```python
from build123d import *

# Parameters (mm, degrees)
F1_DEPTH = 24.13
F2_W     = 15.685529
F2_H     = 20.463388
F3_DEPTH = 11.43
F5_DEPTH = 25.146


with BuildPart() as f1:
    # F0 (on Right) → F1 (new body)
    with BuildSketch(Plane.YZ):
        Polygon((0, 21.47734), (-69.962664, 21.47734), (-69.962664, 2.857499), (-33.644756, 2.857499), (0, 2.857499), align=None)
        Polygon((-33.644756, 2.857499), (-69.962664, 2.857499), (-87.845083, 2.857499), (-87.845083, -17.605888), (-33.644756, -17.605888), align=None)
    extrude(amount=F1_DEPTH)

    # F2 (on Right) → F3 (cut)
    with BuildSketch(Plane.YZ):
        with Locations((-7.842764, 12.16742)):
            Rectangle(F2_W, F2_H)
    extrude(amount=F3_DEPTH, mode=Mode.SUBTRACT)

    # F4 (on Right) → F5 (join)
    with BuildSketch(Plane.YZ):
        Polygon((-0.056833, 21.314132), (-70.019497, 21.314132), (-70.019497, 2.694292), (-33.701589, 2.694292), (-0.056833, 2.694292), align=None)
        Polygon((-33.701589, 2.694292), (-70.019497, 2.694292), (-87.901916, 2.694292), (-87.901916, -17.769095), (-33.701589, -17.769095), align=None)
    extrude(amount=-F5_DEPTH)


solid = f1.part
```
Geometry: final body of the model. Coordinates: model frame, mm. A direction names the side the tool comes from. Coordinates: 2 decimals unless noted, no trailing zeros. Order: outer loops, then holes, each group sorted by start corner. A loop starts at its lowest first (then second) coordinate and runs counter-clockwise, first axis right, second up. Notation, with made-up numbers: M 77,-7.5 L 112,-7.5 A21 cw 112,13.5 Z; hole C 68,-26 d6. An arc over 180 degrees is marked long. Answer in a Markdown table with one row per item. Add a question column.
Q1. Contact query for flat-ended pins moving along their axis: P1, Ø5, axis at x = -3.5, y = -58, coming from the +Z side; P2, Ø8, axis at x = -18.5, z = 15, coming from the +Y side; P3, Ø5, axis at x = -9.5, y = -30, coming from the -Z side. Output: stop coordinate, or through.
Q2. Line query: L1, parallel to Z at x = 11, y = -84; L2, parallel to Y at x = -1, z = -15; L3, parallel to Z at x = -23, y = -19. Output: solid intervals per line, ascending.
Q3. Mould query, pull axis X, two halves, no side actions, for faces 1 (the flat face through (24.13, -45, 2)), 2 (the flat face through (0, -10, 12)), 3 (the flat face through (12, -87.845, -7)), 4 (the flat face through (6, -15.686, 12)). Classes: released by +X, released by -X, zero draft, split by the parting line, or undercut.
Q4. Section query D-D on z = 14.5. Return the cut outline in (x, y), and give its area (3 significant figures).
Q5. Section query B-B on z = 1. Return the cut outline in (x, y).
Q6. Section query A-A on y = -6. Return the cut outline in (x, z), and give its area (3 significant figures).
Q7. Reachability of faces 5 (the flat face through (-12, -79, 2.694)), 6 (the flat face through (11.43, -8, 12)), 7 (the flat face through (12, -61, -17.606)), 8 (the flat face through (15, -21, 2.857)) from +Z, -Z, +X, -X, +Y, -Y: full face, straight path, thin tool, end or side. Return the list, or none.
Q8. Section query C-C on x = 7. Return the cut outline in (y, z), and give its area (3 significant figures).
Completed:
| question | item | result |
|---|---|---|
| 1 | P1 | stops at z = 21.31 |
| 1 | P2 | stops at y = -0.06 |
| 1 | P3 | stops at z = 2.69 |
| 2 | L1 | z = -17.61 to 2.86 |
| 2 | L2 | y = -87.9 to -33.7 |
| 2 | L3 | z = 2.69 to 21.31 |
| 3 | face 1 | released by +X |
| 3 | face 2 | undercut |
| 3 | face 3 | zero draft |
| 3 | face 4 | undercut |
| 4 | outline | M -25.15,-70.02 L 0,-70.02 L 0,-69.96 L 24.13,-69.96 L 24.13,0 L 11.43,0 L 11.43,-15.69 L 0,-15.69 L 0,-0.06 L -25.15,-0.06 Z |
| 4 | area | 3,270 mm2 |
| 5 | outline | M -25.15,-87.9 L 0,-87.9 L 0,-87.85 L 24.13,-87.85 L 24.13,-33.64 L 0,-33.64 L 0,-33.7 L -25.15,-33.7 Z |
| 6 | outline | M -25.15,2.69 L 0,2.69 L 0,21.31 L -25.15,21.31 Z; M 11.43,2.86 L 24.13,2.86 L 24.13,21.48 L 11.43,21.48 Z |
| 6 | area | 705 mm2 |
| 7 | face 5 | +Z, -X, -Y |
| 7 | face 6 | +Z, -Z, +Y |
| 7 | face 7 | -Z, +X, +Y, -Y |
| 7 | face 8 | -Z, +X, +Y |
| 8 | outline | M -87.85,-17.61 L -33.64,-17.61 L -33.64,2.86 L -15.69,2.86 L -15.69,21.48 L -69.96,21.48 L -69.96,2.86 L -87.85,2.86 Z |
| 8 | area | 2,120 mm2 |
